```python
from build123d import *

# Parameters (mm, degrees)
SKETCH1_R               = 1.275
BOSS_EXTRUDE1_DEPTH     = 6.5
SKETCH2_W               = 3.53
SKETCH2_H               = 1.96
BOSS_EXTRUDE2_DEPTH     = 1.3
FILLET1_R               = 0.7
SKETCH3_W               = 3.2
SKETCH3_H               = 0.56
SKETCH3_H_2             = 0.5
BOSS_EXTRUDE3_DEPTH     = 0.9
SKETCH4_W               = 1.2
SKETCH4_H               = 0.56
SKETCH4_H_2             = 0.5
BOSS_EXTRUDE4_DEPTH     = 3.47
FILLET2_R               = 0.59
EXTRU_MINCE1_DEPTH      = 2
EXTRU_MINCE1_DEPTH_BACK = 2


with BuildPart() as part:
    # Sketch1 → Boss-Extrude1 (new body)
    with BuildSketch(Plane(origin=(0, 0, 0), x_dir=(0, 0, -1), z_dir=(1, 0, 0))):
        with BuildLine():
            Line((-9.45, 0), (-6.75, 0))
            Line((-6.75, 0), (-6.75, -0.45))
            Line((-6.75, -0.45), (-2.95, -0.45))
            Line((-2.95, -0.45), (-2.95, 0))
            Line((-2.95, 0), (2.95, 0))
            Line((2.95, 0), (2.95, -0.45))
            Line((2.95, -0.45), (6.75, -0.45))
            Line((6.75, -0.45), (6.75, 0))
            Line((6.75, 0), (9.25, 0))
            ThreePointArc((9.25, 0), (9.603553391, 0.146446609), (9.75, 0.5))
            Line((9.75, 0.5), (9.75, 9.02))
            ThreePointArc((9.75, 9.02), (9.603553391, 9.373553391), (9.25, 9.52))
            Line((9.25, 9.52), (-0.25, 9.52))
            Line((-0.25, 9.52), (-0.25, 10.16))
            Line((-0.25, 10.16), (-9.45, 10.16))
            ThreePointArc((-9.45, 10.16), (-9.803553391, 10.013553391), (-9.95, 9.66))
            Line((-9.95, 9.66), (-9.95, 0.5))
            ThreePointArc((-9.95, 0.5), (-9.803553391, 0.146446609), (-9.45, 0))
        make_face()
        with Locations((-4.85, 2.525)):
            Circle(SKETCH1_R, mode=Mode.SUBTRACT)
        with Locations((4.85, 2.525)):
            Circle(SKETCH1_R, mode=Mode.SUBTRACT)
    extrude(amount=BOSS_EXTRUDE1_DEPTH)

    # Sketch2 → Boss-Extrude2 (add)
    with BuildSketch(Plane(origin=(0, 10.16, 0), x_dir=(1, 0, 0), z_dir=(0, 1, 0))):
        with Locations((3.635, -2.77)):
            Rectangle(SKETCH2_W, SKETCH2_H)
    extrude(amount=BOSS_EXTRUDE2_DEPTH)

    # Fillet1
    fillet1_edges = [part.edges().sort_by_distance(p)[0] for p in [
        (3.635, 11.46, 3.75),
        (3.635, 11.46, 1.79),
    ]]
    fillet(fillet1_edges, radius=FILLET1_R)

    # Sketch3 → Boss-Extrude3 (add)
    with BuildSketch(Plane(origin=(0, 0, 0), x_dir=(-1, 0, 0), z_dir=(0, -1, 0))):
        with Locations((-3.25, -8.27)):
            Rectangle(SKETCH3_W, SKETCH3_H)
        with Locations((-3.25, 0.7)):
            Rectangle(SKETCH3_W, SKETCH3_H_2)
        with Locations((-3.25, 7.9)):
            Rectangle(SKETCH3_W, SKETCH3_H_2)
    extrude(amount=BOSS_EXTRUDE3_DEPTH)

    # Sketch4 → Boss-Extrude4 (add)
    with BuildSketch(Plane(origin=(0, -0.9, 0), x_dir=(-1, 0, 0), z_dir=(0, -1, 0))):
        with Locations((-3.25, -8.27)):
            Rectangle(SKETCH4_W, SKETCH4_H)
        with Locations((-3.25, 0.7)):
            Rectangle(SKETCH4_W, SKETCH4_H_2)
        with Locations((-3.25, 7.9)):
            Rectangle(SKETCH4_W, SKETCH4_H_2)
    extrude(amount=BOSS_EXTRUDE4_DEPTH)

    # Fillet2
    fillet2_edges = [part.edges().sort_by_distance(p)[0] for p in [
        (2.65, -4.37, 8.27),
        (3.85, -4.37, 8.27),
        (2.65, -4.37, -0.7),
        (3.85, -4.37, -0.7),
        (3.85, -4.37, -7.9),
        (2.65, -4.37, -7.9),
    ]]
    fillet(fillet2_edges, radius=FILLET2_R)

    # Esquisse1 → Extru.-Mince1 (add, two sides)
    with BuildSketch(Plane(origin=(3.2, 0, 0), x_dir=(0, 0, -1), z_dir=(1, 0, 0))) as extru_mince1_sk:
        with BuildLine():
            Line((-7.25, 10.16), (-7.25, 10.688783991))
            ThreePointArc((-7.25, 10.688783991), (-7.129827698, 11.013946904), (-6.82707632, 11.182807513))
            Line((-6.82707632, 11.182807513), (8.981676404, 13.649249751))
            ThreePointArc((8.981676404, 13.649249751), (9.04222668, 13.683021873), (9.06626114, 13.748054456))
            Line((9.06626114, 13.748054456), (9.06626114, 14.573737504))
            ThreePointArc((9.06626114, 14.573737504), (10.36626114, 15.873737504), (11.66626114, 14.573737504))
            Line((11.66626114, 14.573737504), (11.66626114, 13.717657457))
            Line((11.66626114, 13.717657457), (11.36616114, 13.717657457))
            Line((11.36616114, 13.717657457), (11.36616114, 14.573737504))
            ThreePointArc((11.36616114, 14.573737504), (10.36626114, 15.573637504), (9.36636114, 14.573737504))
            Line((9.36636114, 14.573737504), (9.36636114, 13.748054456))
            ThreePointArc((9.36636114, 13.748054456), (9.270199264, 13.487859093), (9.027937611, 13.352736833))
            Line((9.027937611, 13.352736833), (-6.780815113, 10.886294595))
            ThreePointArc((-6.780815113, 10.886294595), (-6.901855114, 10.818784123), (-6.9499, 10.688783991))
            Line((-6.9499, 10.688783991), (-6.9499, 10.16))
            Line((-6.9499, 10.16), (-7.25, 10.16))
        make_face()
    extrude(amount=EXTRU_MINCE1_DEPTH)
    extrude(extru_mince1_sk.sketch, amount=-EXTRU_MINCE1_DEPTH_BACK)


solid = part.part
```
Work out the finished part from the listing and answer in its coordinate system (mm). A direction names the side the tool comes from. Give positions to 0.01 mm unless a question says otherwise; leave off trailing zeros. Order: outer loops, then holes, each group sorted by start corner. A loop starts at its lowest first (then second) coordinate and runs counter-clockwise, first axis right, second up. Notation, with made-up numbers: (47.25, 78) - (87.25, 78) arc R22 cw to (87.25, 95) - close; hole circle Ø7 at (7.25, -8). An arc over 180 degrees is marked (long way). One line per item, written item: value. Start each with the question number.
1. Each of these flat-tipped pins is pushed along its axis until it touches: pin 1 Ø0.6 at (y, z) = (-0.5, -8) entering from -X; pin 2 Ø1 at (x, z) = (2, 3) entering from +Y; pin 3 Ø1.8 at (x, z) = (4, -1) entering from -Y; pin 4 Ø6 at (y, z) = (13.5, -1) entering from +X. Where does it stop, or does it pass through?
2. Section B-B, the plane z = 4.85 is taken. Write down the section's boundary in (x, y), then the cut area to 3 significant figures.
3. Section A-A, the plane y = -2.25 is taken. Write down the section's boundary in (x, z), then the cut area to 3 significant figures.
4. Consider line 1 (Y direction, x = 2.5, z = 4.5); line 2 (Z direction, x = 3.75, y = 3.5); line 3 (Z direction, x = 3, y = 13.75). Determine where each line is inside the solid, lowest interval first.
5. For a pull along Z with two mould halves and no side action, classify faces 1 (the face through (3, 14, -9.066)), 2 (the face through (3.228, 15.573, -10.388)), 3 (the face through (3, 9.52, -5)), 4 (the face through (3, 5, -9.75)) as released by +Z, released by -Z, zero draft, split by the parting line, or undercut.
6. Which of the six approach directions +Z, -Z, +X, -X, +Y, -Y give full straight-line access (tool end or side, diameter ignored) to faces 5 (the face through (6.5, 5, 0)), 6 (the face through (3, -2, 8.55)), 7 (the face through (3, -2, -8.15)), 8 (the face through (3, -2, -0.45)), 9 (the face through (5.4, 11, 3))?
7. Section C-C, the plane y = 5 is taken. Write down the section's boundary in (x, z), then the cut area to 3 significant figures.
Filled sheet:
1. pin 1: x = 1.65
1. pin 2: y = 11.86
1. pin 3: y = -4.37
1. pin 4: x = 5.2
2. outline: (0, -0.45) - (6.5, -0.45) - (6.5, 1.25) - (0, 1.25) - close; (0, 3.8) - (6.5, 3.8) - (6.5, 10.16) - (0, 10.16) - close; (1.2, 11.19) - (5.2, 11.19) - (5.2, 11.49) - (1.2, 11.49) - close
2. area: 53.6 mm²
3. outline: (2.65, -8.15) - (3.85, -8.15) - (3.85, -7.65) - (2.65, -7.65) - close; (2.65, -0.95) - (3.85, -0.95) - (3.85, -0.45) - (2.65, -0.45) - close; (2.65, 7.99) - (3.85, 7.99) - (3.85, 8.55) - (2.65, 8.55) - close
3. area: 1.87 mm²
4. line 1: -0.45 to 1.3, 3.75 to 10.16, 11.24 to 11.55
4. line 2: -9.75 to -5.67, -4.03 to 4.03, 5.67 to 9.95
4. line 3: -11.67 to -11.37, -9.37 to -9.07
5. face 1: released by +Z
5. face 2: undercut
5. face 3: zero draft
5. face 4: released by -Z
6. face 5: +Z, -Z, +X, +Y, -Y
6. face 6: +Z, +X, -X, -Y
6. face 7: -Z, +X, -X, -Y
6. face 8: +X, -X, -Y
6. face 9: +Z, -Z, +X, +Y
7. outline: (0, -9.75) - (6.5, -9.75) - (6.5, 9.95) - (0, 9.95) - close
7. area: 128 mm²
